Design review of the part built by this model. Coordinates are the model's own, in mm. A direction names the side the tool comes from. Coordinates: 2 decimals unless noted, no trailing zeros. Loops run counter-clockwise (first coordinate to the right, second up) from the corner with the lowest first, then second, coordinate; pieces in that order, holes last. Notation, with made-up numbers: (36, -36.75) - (94, -36.75) arc R22 cw to (94, -12.75) - close; hole circle Ø9 at (9.25, 3.5). An arc over 180 degrees is marked (long way). Return JSON: item names as keys, results as strings. Group by question number.
from build123d import *

# Parameters (mm, degrees)
SKETCH1_R            = 28.1
SKETCH1_R_2          = 21.1
BOSS_EXTRUDE1_DEPTH  = 4.5
SKETCH2_R            = 28.1
SKETCH2_R_2          = 18.6
BOSS_EXTRUDE2_DEPTH  = 3
M3_CLEARANCE_HOLE1_D = 3.2
CUT_EXTRUDE1_DEPTH   = 2
CIRPATTERN1_COUNT    = 6
CHAMFER1_SIZE        = 2
CHAMFER1_SIZE_2      = 5.494954839


with BuildPart() as part:
    # Sketch1 → Boss-Extrude1 (new body)
    with BuildSketch(Plane.XY):
        Circle(SKETCH1_R)
        Circle(SKETCH1_R_2, mode=Mode.SUBTRACT)
    extrude(amount=BOSS_EXTRUDE1_DEPTH)

    # Sketch2 → Boss-Extrude2 (add)
    with BuildSketch(Plane.XY.offset(4.5)):
        Circle(SKETCH2_R)
        Circle(SKETCH2_R_2, mode=Mode.SUBTRACT)
    extrude(amount=BOSS_EXTRUDE2_DEPTH)

    # M3 Clearance Hole1 (through all)
    with Locations(Plane(origin=(0, 0, 0), x_dir=(-1, 0, 0), z_dir=(0, 0, -1))):
        with Locations((0, 24.6)):
            m3_clearance_hole1 = Hole(M3_CLEARANCE_HOLE1_D / 2)

    # Sketch5 → Cut-Extrude1 (cut)
    with BuildSketch(Plane.XY.offset(7.5)):
        Polygon((-1.645448267, 27.45), (1.645448267, 27.45), (3.290896534, 24.6), (1.645448267, 21.75), (-1.645448267, 21.75), (-3.290896534, 24.6), align=None)
    cut_extrude1 = extrude(amount=-CUT_EXTRUDE1_DEPTH, mode=Mode.SUBTRACT)

    # CirPattern1: M3 Clearance Hole1, Cut-Extrude1 ×6 about axis
    cirpattern1_axis = Axis((0, 0, 0), (0, 0, 1))
    add([m3_clearance_hole1.rotate(cirpattern1_axis, i * 360 / CIRPATTERN1_COUNT) for i in range(1, CIRPATTERN1_COUNT)], mode=Mode.SUBTRACT)
    add([cut_extrude1.rotate(cirpattern1_axis, i * 360 / CIRPATTERN1_COUNT) for i in range(1, CIRPATTERN1_COUNT)], mode=Mode.SUBTRACT)

    # Chamfer1
    # the kernel refuses this chamfer: 5.494954839, 2 mm, written as the material it takes off along each edge
    with BuildSketch(Plane(origin=(0, 0, 7.5), x_dir=(1, 0, 0), z_dir=(0, -1, 0))) as chamfer1_piece_1:
        Polygon((18.6 + CHAMFER1_SIZE, 0), (18.6, -CHAMFER1_SIZE_2), (18.6, 0), align=None)
    revolve(axis=Axis((0, 0, 7.5), (0, 0, 1)), mode=Mode.SUBTRACT)


solid = part.part
Item 1: Add section C-C (z = 3.75). State the section outline as (x, y) points, then the cut area to 3 significant figures.
Item 2: To check wall thickness, follow line 1 (Y direction, x = 0, z = 2); line 2 (X direction, y = 15, z = 6.75); line 3 (Y direction, x = -6, z = 5.75). State the ranges of each line that lie inside material, in increasing order. Write a range as from..to.
Item 3: For P1, Ø12, axis at x = -9.5, y = 8.5, coming from the -Z side; P2, Ø4, axis at x = -21.3, y = -12.3, coming from the +Z side; P3, Ø1.5, axis at y = -12.5, z = 4.5, coming from the -X side; P4, Ø2, axis at x = 22, z = 7, coming from the +Y side, all flat-tipped, find the tip position at first contact; note any pin that passes through.
Item 4: For faces 1 (the face through (21, -9.45, 7)), 2 (the face through (0.208, -26.186, 2.788)), list the 3-axis set-ups (+Z, -Z, +X, -X, +Y, -Y) from which the entire face can be reached by the end or side of a thin tool; tool diameter is ignored.
Item 5: Add section A-A (y = 0). State the section outline as (x, z) points, then the cut area to 3 significant figures.
Item 6: Draft analysis for pull direction Y (two halves, no side actions). For faces 3 (the face through (-4, -21, 0)), 4 (the face through (-2.48, 26.005, 6.514)), 5 (the face through (-6.092, -27.432, 3.698)), state which applies: pulls with the +Y half, pulls with the -Y half, needs draft (parallel to the pull), parting line crosses it, or undercut.
Item 7: Add section B-B (x = 0). State the section outline as (y, z) points, then the cut area to 3 significant figures.
Answers below:
{
 "1": {"outline": "circle Ø56.2 at (0, 0); hole circle Ø3.2 at (-21.3, -12.3); hole circle Ø3.2 at (-21.3, 12.3); hole circle Ø42.2 at (0, 0); hole circle Ø3.2 at (0, -24.6); hole circle Ø3.2 at (0, 24.6); hole circle Ø3.2 at (21.3, -12.3); hole circle Ø3.2 at (21.3, 12.3)", "area": "1,030 mm^2"},
 "2": {"line 1": "y = -28.1..-26.2, -23..-21.1, 21.1..23, 26.2..28.1", "line 2": "x = -23.76..-23.04, -19.57..-13.72, 13.72..19.57, 23.04..23.76", "line 3": "y = -27.45..-19.04, 19.04..27.45"},
 "3": {"P1": "passes through", "P2": "stops at z = 5.5", "P3": "stops at x = -25.53", "P4": "stops at y = 18.67"},
 "4": {"face 1": "+Z", "face 2": "+Z, -Z"},
 "5": {"outline": "(-28.1, 0) - (-21.1, 0) - (-21.1, 4.5) - (-19.51, 4.5) - (-20.6, 7.5) - (-28.1, 7.5) - close; (19.51, 4.5) - (21.1, 4.5) - (21.1, 0) - (28.1, 0) - (28.1, 7.5) - (20.6, 7.5) - close", "area": "111 mm^2"},
 "6": {"face 3": "needs draft", "face 4": "undercut", "face 5": "parting line crosses it"},
 "7": {"outline": "(-28.1, 0) - (-26.2, 0) - (-26.2, 5.5) - (-27.45, 5.5) - (-27.45, 7.5) - (-28.1, 7.5) - close; (-23, 0) - (-21.1, 0) - (-21.1, 4.5) - (-19.51, 4.5) - (-20.6, 7.5) - (-21.75, 7.5) - (-21.75, 5.5) - (-23, 5.5) - close; (19.51, 4.5) - (21.1, 4.5) - (21.1, 0) - (23, 0) - (23, 5.5) - (21.75, 5.5) - (21.75, 7.5) - (20.6, 7.5) - close; (26.2, 0) - (28.1, 0) - (28.1, 7.5) - (27.45, 7.5) - (27.45, 5.5) - (26.2, 5.5) - close", "area": "53.3 mm^2"}
}
